from build123d import *

# Parameters (mm, degrees)
ESQUISSE1_W                                 = 145.148196
ESQUISSE1_H                                 = 60
BOSS_EXTRU_1_DEPTH                          = 1.5
BOSS_EXTRU_2_DEPTH                          = 2
FRAISAGE_POUR_VIS_T_TE_FRAIS_E_M31_AT_COUNT = 2
FRAISAGE_POUR_VIS_T_TE_FRAIS_E_M31_AT_PITCH = 52
FRAISAGE_POUR_VIS_T_TE_FRAIS_E_M31_2_COUNT  = 2
FRAISAGE_POUR_VIS_T_TE_FRAIS_E_M31_2_PITCH  = 135.572178
FRAISAGE_POUR_VIS_T_TE_FRAIS_E_M31_3_COUNT  = 2
FRAISAGE_POUR_VIS_T_TE_FRAIS_E_M31_3_PITCH  = 145.20267025
ENL_V_MAT_EXTRU_1_DEPTH                     = 79.608203774
ENL_V_MAT_EXTRU_1_DEPTH_BACK                = 79.608203774
ESQUISSE6_W                                 = 24
ESQUISSE6_H                                 = 6
CONG_1_R                                    = 3


with BuildPart() as part:
    # Esquisse1 → Boss.-Extru.1 (new body)
    with BuildSketch(Plane.XY):
        Rectangle(ESQUISSE1_W, ESQUISSE1_H)
    extrude(amount=BOSS_EXTRU_1_DEPTH)

    # Esquisse2 → Boss.-Extru.2 (add)
    with BuildSketch(Plane(origin=(0, 0, 0), x_dir=(-1, 0, 0), z_dir=(0, 0, -1))):
        with BuildLine():
            Line((-71.374098, -16.8), (-71.374098, 16.8))
            ThreePointArc((-71.374098, 16.8), (-64.303030188, 19.728932188), (-61.374098, 26.8))
            Line((-61.374098, 26.8), (61.374098, 26.8))
            ThreePointArc((61.374098, 26.8), (64.303030188, 19.728932188), (71.374098, 16.8))
            Line((71.374098, 16.8), (71.374098, -16.8))
            ThreePointArc((71.374098, -16.8), (64.303030188, -19.728932188), (61.374098, -26.8))
            Line((61.374098, -26.8), (-61.374098, -26.8))
            ThreePointArc((-61.374098, -26.8), (-64.303030188, -19.728932188), (-71.374098, -16.8))
        make_face()
    extrude(amount=BOSS_EXTRU_2_DEPTH)

    # Esquisse5 → Fraisage pour vis à tête fraisée M31 (revolve, cut)
    with BuildSketch(Plane(origin=(-68.574098, 26, 1.5), x_dir=(0, -1, 0), z_dir=(1, 0, 0))):
        Polygon((0, 0), (0, 1.5), (1.7, 1.5), (1.7, 1.45), (3.15, 0), align=None)
    fraisage_pour_vis_t_te_frais_e_m31 = revolve(axis=Axis((-68.574098, 26, 7.85), (0, 0, -1)), mode=Mode.SUBTRACT)

    # Fraisage pour vis à tête fraisée M31 at: Fraisage pour vis à tête fraisée M31 ×2
    with Locations(*[(0, -i * FRAISAGE_POUR_VIS_T_TE_FRAIS_E_M31_AT_PITCH, 0) for i in range(1, FRAISAGE_POUR_VIS_T_TE_FRAIS_E_M31_AT_COUNT)]):
        add(fraisage_pour_vis_t_te_frais_e_m31, mode=Mode.SUBTRACT)

    # Fraisage pour vis _ t_te frais_e M31 2: Fraisage pour vis à tête fraisée M31 ×2
    with Locations(*[(i * FRAISAGE_POUR_VIS_T_TE_FRAIS_E_M31_2_PITCH, 0, 0) for i in range(1, FRAISAGE_POUR_VIS_T_TE_FRAIS_E_M31_2_COUNT)]):
        add(fraisage_pour_vis_t_te_frais_e_m31, mode=Mode.SUBTRACT)

    # Fraisage pour vis _ t_te frais_e M31 3: Fraisage pour vis à tête fraisée M31 ×2
    with Locations(*[Vector(0.9336755155176905, -0.35812013588009123, 0) * (i * FRAISAGE_POUR_VIS_T_TE_FRAIS_E_M31_3_PITCH) for i in range(1, FRAISAGE_POUR_VIS_T_TE_FRAIS_E_M31_3_COUNT)]):
        add(fraisage_pour_vis_t_te_frais_e_m31, mode=Mode.SUBTRACT)

    # Esquisse6 → Enlèv. mat.-Extru.1 (cut, two sides: drawn at the far end of the back side and taken through both)
    with BuildSketch(Plane.XY.offset(1.5).offset(-ENL_V_MAT_EXTRU_1_DEPTH_BACK)):
        with Locations((-40.574098, 27)):
            Rectangle(ESQUISSE6_W, ESQUISSE6_H)
    extrude(amount=ENL_V_MAT_EXTRU_1_DEPTH + ENL_V_MAT_EXTRU_1_DEPTH_BACK, mode=Mode.SUBTRACT)

    # Congé1
    cong_1_edges = [part.edges().sort_by_distance(p)[0] for p in [
        (-28.574098, 30, 0.75),
        (-28.574098, 24, -0.25),
        (-52.574098, 30, 0.75),
        (-52.574098, 24, -0.25),
    ]]
    fillet(cong_1_edges, radius=CONG_1_R - 0.0001)  # a hair under: the kernel refuses the full size


solid = part.part
The model under review builds one solid part; all positions refer to its coordinate system, in mm. A direction names the side the tool comes from. Round coordinates to 2 decimals unless told otherwise and drop trailing zeros. Loops run counter-clockwise (first coordinate to the right, second up) from the corner with the lowest first, then second, coordinate; pieces in that order, holes last. Notation, with made-up numbers: (-29, 65.5) - (-6, 65.5) arc R14 cw to (-6, 80.5) - close; hole circle Ø7 at (45.25, 14.5). An arc over 180 degrees is marked (long way). Use CSV: the item, a comma, the result in double quotes.
(1) The part is to be moulded in two halves that separate along X. For faces 6 (the cylindrical face through (-53.476, 29.145, 0.76)), 7 (the cylindrical face through (-64.38, -19.65, -0.99)), 8 (the flat face through (0, 27, 0)), say which applies: pulls with the +X half, pulls with the -X half, needs draft (parallel to the pull), parting line crosses it, or undercut.
Working result:
face 6,"undercut"
face 7,"pulls with the -X half"
face 8,"needs draft"
(2) Clearance check with flat-ended pins moving along their axes: P1, Ø2, axis at x = 25.5, z = -1.5, coming from the -Y side; P2, Ø2.5, axis at x = 67, y = -26, coming from the -Z side; P3, Ø0.6, axis at x = 8, z = -1.5, coming from the +Y side; P4, Ø0.6, axis at y = 3.5, z = -1.5, coming from the -X side. State where each tip first meets the part, or that it passes through.
Working result:
P1,"stops at y = -26.8"
P2,"passes through"
P3,"stops at y = 26.8"
P4,"stops at x = -71.37"
(3) Machinability: for faces 1 (the cylindrical face through (64.38, 19.65, -0.99)), 2 (the cylindrical face through (-29.43, 24.9, -0.23)), 3 (the flat face through (-1, 0, -2)), 4 (the cylindrical face through (-64.226, 19.807, -0.986)), 5 (the flat face through (-1, 0, 1.5)), which of the approach directions +Z, -Z, +X, -X, +Y, -Y give a long, thin tool a straight path to every point of the face, cutting with its end or side? Answer none if there is none.
Working result:
face 1,"-Z, +X, +Y"
face 2,"+Z, -Z, +Y"
face 3,"-Z, +X, -X, +Y, -Y"
face 4,"-Z, -X, +Y"
face 5,"+Z, +X, -X, +Y, -Y"
(4) Take a section at B-B, the plane z = 0.8. State how many separate pieces and enclosed holes the cut face has, plus the area to 3 significant figures.
Working result:
separate pieces,"1"
enclosed holes,"4"
area,"8,490 mm^2"
(5) Take a section at C-C, the plane x = -63. Give the boundary of the cut face in (y, z).
Working result:
outline,"(-30, 0) - (-21.33, 0) - (-21.33, -2) - (21.33, -2) - (21.33, 0) - (30, 0) - (30, 1.5) - (-30, 1.5) - close"
(6) For line 1 (Y direction, x = 27, z = -1); line 2 (X direction, y = 26, z = 0.05); line 3 (Y direction, x = -38, z = -0.4), list the stretches that pass through material, from the lowest coordinate up.
Working result:
line 1,"y = -26.8 to 26.8"
line 2,"x = -72.57 to -70.27, -66.87 to -52.4, -28.75 to 65.3, 68.7 to 72.57"
line 3,"y = -26.8 to 24"
(7) Take a section at D-D, the plane x = -42. Give the boundary of the cut face in (y, z), plus the area to 3 significant figures.
Working result:
outline,"(-30, 0) - (-26.8, 0) - (-26.8, -2) - (24, -2) - (24, 1.5) - (-30, 1.5) - close"
area,"183 mm^2"
(8) Take a section at A-A, the plane x = 20.5. Give the boundary of the cut face in (y, z).
Working result:
outline,"(-30, 0) - (-26.8, 0) - (-26.8, -2) - (26.8, -2) - (26.8, 0) - (30, 0) - (30, 1.5) - (-30, 1.5) - close"
